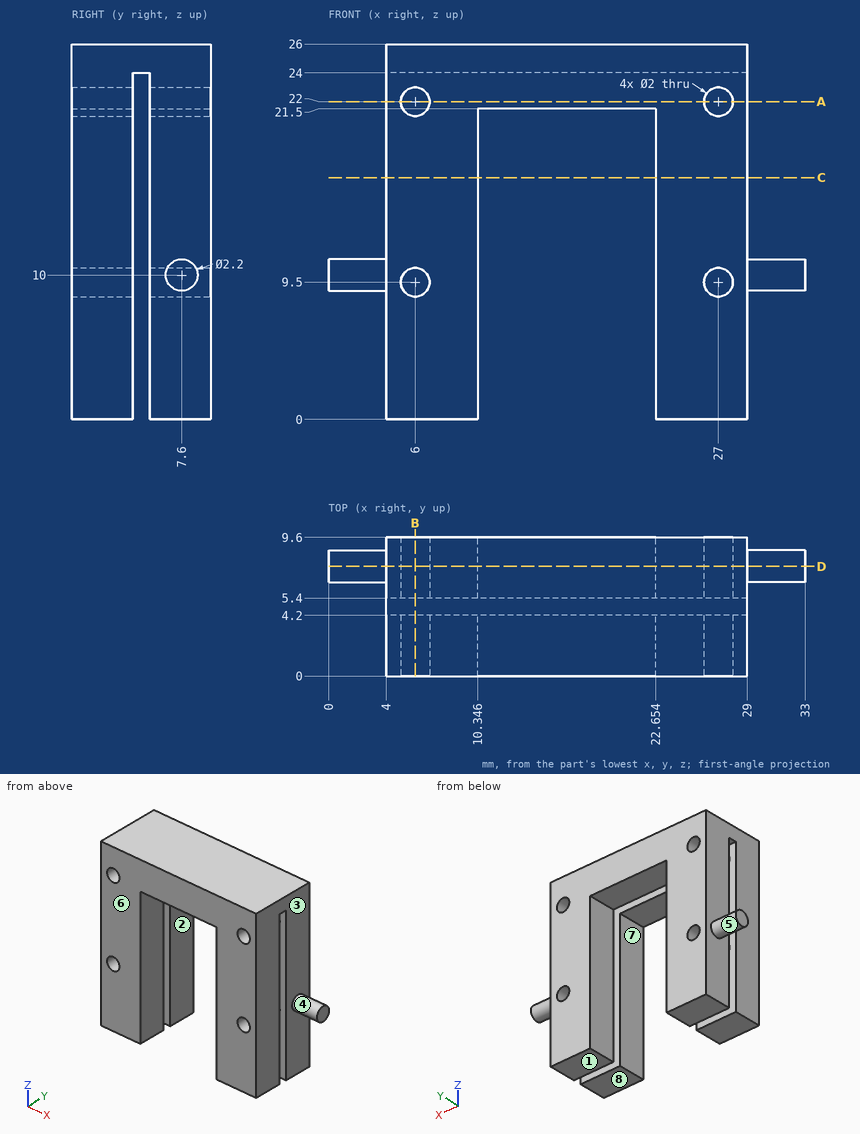
Drawing for the job (mm, zero at the part's lowest x, y, z). A direction names the side the tool comes from. Coordinates: 2 decimals unless noted, no trailing zeros. Loops run counter-clockwise (first coordinate to the right, second up) from the corner with the lowest first, then second, coordinate; pieces in that order, holes last. Notation, with made-up numbers: (20, 65.25) - (28, 65.25) arc R29 ccw to (28, 101.25) - close; hole circle Ø7 at (-11, 46.5). An arc over 180 degrees is marked (long way). Return JSON: item names as keys, results as strings.
1. Band-saw the part on A-A (z = 22). Give the cut face in (x, y), and give its area (3 significant figures).
Result:
{"outline": "(4, 0) - (5, 0) - (5, 4.2) - (4, 4.2) - close; (4, 5.4) - (5, 5.4) - (5, 9.6) - (4, 9.6) - close; (7, 0) - (26, 0) - (26, 4.2) - (7, 4.2) - close; (7, 5.4) - (26, 5.4) - (26, 9.6) - (7, 9.6) - close; (28, 0) - (29, 0) - (29, 4.2) - (28, 4.2) - close; (28, 5.4) - (29, 5.4) - (29, 9.6) - (28, 9.6) - close", "area": "176 mm2"}
2. Band-saw the part on C-C (z = 16.75). Give the cut face in (x, y), and give its area (3 significant figures).
Result:
{"outline": "(4, 0) - (10.35, 0) - (10.35, 4.2) - (4, 4.2) - close; (4, 5.4) - (10.35, 5.4) - (10.35, 9.6) - (4, 9.6) - close; (22.65, 0) - (29, 0) - (29, 4.2) - (22.65, 4.2) - close; (22.65, 5.4) - (29, 5.4) - (29, 9.6) - (22.65, 9.6) - close", "area": "107 mm2"}
3. Band-saw the part on B-B (x = 6). Give the cut face in (y, z), and give its area (3 significant figures).
Result:
{"outline": "(0, 0) - (4.2, 0) - (4.2, 8.5) - (0, 8.5) - close; (0, 10.5) - (4.2, 10.5) - (4.2, 21) - (0, 21) - close; (0, 23) - (4.2, 23) - (4.2, 24) - (5.4, 24) - (5.4, 23) - (9.6, 23) - (9.6, 26) - (0, 26) - close; (5.4, 0) - (9.6, 0) - (9.6, 8.5) - (5.4, 8.5) - close; (5.4, 10.5) - (9.6, 10.5) - (9.6, 21) - (5.4, 21) - close", "area": "187 mm2"}
4. Drop flat-ended pins along their axis: pin 1 (3.5 mm diameter, centred on x = 14.5, y = 3, fed in from -Z); pin 2 (5 mm diameter, centred on y = 8, z = 21, fed in from +X). Give the stop position or say it passes through.
Result:
{"pin 1": "stops at z = 21.5", "pin 2": "stops at x = 29"}
5. Band-saw the part on D-D (y = 7.6). Give the cut face in (x, z).
Result:
{"outline": "(0, 8.9) - (4, 8.9) - (4, 0) - (10.35, 0) - (10.35, 21.5) - (22.65, 21.5) - (22.65, 0) - (29, 0) - (29, 8.9) - (33, 8.9) - (33, 11.1) - (29, 11.1) - (29, 26) - (4, 26) - (4, 11.1) - (0, 11.1) - close; hole circle Ø2 at (6, 9.5); hole circle Ø2 at (6, 22); hole circle Ø2 at (27, 9.5); hole circle Ø2 at (27, 22)"}
6. Probe L1, parallel to Z at x = 27, y = 0.9; L2, parallel to X at y = 1.6, z = 22; L3, parallel to X at y = 7, z = 9.5. List the from-to ranges inside material, lowest first. Write a range as from..to.
Result:
{"L1": "z = 0..8.5, 10.5..21, 23..26", "L2": "x = 4..5, 7..26, 28..29", "L3": "x = 0..5, 7..10.35, 22.65..26, 28..33"}
7. 3-axis set-ups, long thin cutter, end or side, ignore diameter. For the marked faces 4, 5, 6, 7 and 8: which of +Z, -Z, +X, -X, +Y, -Y reach the whole face in a straight line?
Result:
{"face 4": "+X", "face 5": "-X", "face 6": "+Z, -Z, +X, -X, -Y", "face 7": "-Z, +Y, -Y", "face 8": "-Z, +X, -X, +Y, -Y"}
8. Mould opens along X. For the marked faces 1, 2 and 3 say: released by +X, released by -X, zero draft, split by the parting line, or undercut.
Result:
{"face 1": "zero draft", "face 2": "undercut", "face 3": "released by +X"}
